from build123d import *

# Parameters (mm, degrees)
DOWELSUPPORT_DEPTH          = 1.905
DOWELSUPPORT_DEPTH_BACK     = 1.27
SKETCH3_R                   = 3.81
SKETCH5_W                   = 6.35
SKETCH5_H                   = 44.45
SLIDERDOWELSUPPORT_DEPTH    = 1.27
SKETCH17_R                  = 1.549999948
CUT_EXTRUDE1_DEPTH          = 19.685
CUT_EXTRUDE2_DEPTH          = 36.118212712
CUT_EXTRUDE2_DEPTH_BACK     = 36.118212712
SKETCH18_W                  = 1.27
SKETCH18_H                  = 25.4
LPATTERN1_COUNT             = 2
LPATTERN1_PITCH             = 25.4
LATERALSUPPORT_DEPTH        = 1.27
SKETCH8_W                   = 6.35
SKETCH8_H                   = 3
TABSUPPORT_DEPTH            = 1.27
STRINGDOWELSUPPORT_START    = -1.27
STRINGDOWELSUPPORT_DEPTH    = 5.715
INTERSUPPORT_DEPTH          = 1.27
SKETCH10_W                  = 6.35
SKETCH10_H                  = 3
TABBASE_DEPTH               = 1.27
SKETCH12_W                  = 6.35
SKETCH12_H                  = 3
TABDRAFT_DEPTH              = 1.73
TABDRAFT_DRAFT              = 5
TABDRAFT_PROFILE_2_DEPTH    = 1.73
TABDRAFT_PROFILE_2_DRAFT    = 5
STRINGDOWELHOLES_DEPTH      = 48.707819409
STRINGDOWELHOLES_DEPTH_BACK = 1.524
SKETCH14_R                  = 1.600000102
PULLEYDOWELHOLE_DEPTH       = 2.921
FILLET1_R                   = 6.35


with BuildPart() as part:
    # Sketch3 → DowelSupport (new, two sides: drawn at the far end of the back side and taken through both)
    with BuildSketch(Plane(origin=(0, 0, 0), x_dir=(0, 0, -1), z_dir=(1, 0, 0)).offset(-DOWELSUPPORT_DEPTH_BACK)):
        with Locations((0, 30.95625)):
            Circle(SKETCH3_R)
    extrude(amount=DOWELSUPPORT_DEPTH + DOWELSUPPORT_DEPTH_BACK)

    # Sketch8 → TabSupport (add, symmetric)
    with BuildSketch(Plane(origin=(0, 0, 0), x_dir=(0, 0, -1), z_dir=(1, 0, 0))):
        with Locations((0, 27.94)):
            Rectangle(SKETCH8_W, SKETCH8_H)
        with Locations((-12.7, 27.94)):
            Rectangle(SKETCH8_W, SKETCH8_H)
    extrude(amount=TABSUPPORT_DEPTH, both=True)


with BuildPart() as body_2:
    # Sketch5 → SliderDowelSupport (new, symmetric)
    with BuildSketch(Plane(origin=(0, 0, 0), x_dir=(0, 0, -1), z_dir=(1, 0, 0))):
        Rectangle(SKETCH5_W, SKETCH5_H)
    extrude(amount=SLIDERDOWELSUPPORT_DEPTH, both=True)

    # Sketch17 → Cut-Extrude1 (cut, symmetric)
    with BuildSketch(Plane(origin=(0, 0, 0), x_dir=(1, 0, 0), z_dir=(0, 1, 0))):
        with Locations((0.482000052, 0)):
            Circle(SKETCH17_R)
        with BuildLine():
            Line((2.032, 0), (2.032, 1.399999994))
            Line((2.032, 1.399999994), (1.147206678, 1.399999994))
            ThreePointArc((1.147206678, 1.399999994), (1.792261491, 0.828078983), (2.032, 0))
        make_face()
        with BuildLine():
            Line((2.032, -1.399999994), (2.032, 0))
            ThreePointArc((2.032, 0), (1.792261491, -0.828078983), (1.147206678, -1.399999994))
            Line((1.147206678, -1.399999994), (2.032, -1.399999994))
        make_face()
    extrude(amount=CUT_EXTRUDE1_DEPTH, both=True, mode=Mode.SUBTRACT)

    # Sketch18 → Cut-Extrude2 (cut, two sides: drawn at the far end of the back side and taken through both)
    with BuildSketch(Plane.ZY.offset(1.27).offset(-CUT_EXTRUDE2_DEPTH_BACK)):
        Rectangle(SKETCH18_W, SKETCH18_H)
    extrude(amount=CUT_EXTRUDE2_DEPTH + CUT_EXTRUDE2_DEPTH_BACK, mode=Mode.SUBTRACT)


with BuildPart() as lpattern1_1:
    # LPattern1: pattern copy
    add(body_2.part.moved(Location(Vector(0, 0, 1) * (1 * LPATTERN1_PITCH))))


with BuildPart() as body_4:
    # Sketch6 → LateralSupport (new, symmetric)
    with BuildSketch(Plane(origin=(0, 0, 0), x_dir=(0, 0, -1), z_dir=(1, 0, 0))):
        Polygon((7.392863577, 33.391434671), (5.805363577, 36.141065329), (8.169612929, 37.506065329), (9.523465192, 37.701124423), (10.602965192, 35.831375577), (9.757112929, 34.756434671), align=None)
    extrude(amount=LATERALSUPPORT_DEPTH, both=True)


with BuildPart() as tabsupport_piece_1:
    # of the separate pieces the step leaves, piece 1, a body of its own (tabsupport_pieces)
    add(part.part.solids().sort_by_distance((0, 30.95625, -3.81))[0])


with BuildPart() as tabsupport_piece_2:
    # of the separate pieces the step leaves, piece 2, a body of its own (tabsupport_pieces)
    add(part.part.solids().sort_by_distance((-1.27, 26.44, 9.525))[0])

    # Sketch15 → StringDowelSupport (add)
    with BuildSketch(Plane(origin=(0, 0, 0), x_dir=(0, 0, -1), z_dir=(1, 0, 0)).offset(STRINGDOWELSUPPORT_START)):
        with BuildLine():
            Line((-14.4145, 30.226), (-10.9855, 30.226))
            ThreePointArc((-10.9855, 30.226), (-8.6995, 27.94), (-10.9855, 25.654))
            Line((-10.9855, 25.654), (-14.4145, 25.654))
            ThreePointArc((-14.4145, 25.654), (-16.7005, 27.94), (-14.4145, 30.226))
        make_face()
    extrude(amount=STRINGDOWELSUPPORT_DEPTH)


with BuildPart() as body_2_1:
    add(body_2.part)

    add(lpattern1_1.part)  # InterSupport merges LPattern1_1

    add(body_4.part)  # InterSupport merges body 4

    add(tabsupport_piece_1.part)  # InterSupport merges TabSupport piece 1

    add(tabsupport_piece_2.part)  # InterSupport merges TabSupport piece 2
    # Sketch7 → InterSupport (add, symmetric)
    with BuildSketch(Plane(origin=(0, 0, 0), x_dir=(0, 0, -1), z_dir=(1, 0, 0))):
        Polygon((5.170363577, 37.240917591), (8.027863577, 32.291582409), (1.42875, 28.481582409), (-1.42875, 33.430917591), align=None)
        Polygon((-3.175, 15.875), (-3.175, 22.225), (3.175, 22.225), (3.175, 26.44), (0.923046602, 28.251940251), (-0.923046602, 33.660559749), (-10.9855, 30.226), (-14.4145, 30.226), (-15.109807039, 29.269115541), (-28.575, 22.225), (-22.225, 22.225), (-22.225, 0), (-3.175, 0), align=None)
    extrude(amount=INTERSUPPORT_DEPTH, both=True)

    # Sketch10 → TabBase (add)
    with BuildSketch(Plane.ZY.offset(1.27)):
        with Locations((0, 27.94)):
            Rectangle(SKETCH10_W, SKETCH10_H)
        with Locations((12.7, 27.94)):
            Rectangle(SKETCH10_W, SKETCH10_H)
    extrude(amount=TABBASE_DEPTH)


with BuildPart() as tabdraft_tool:
    # Sketch12 → TabDraft (with draft: the straight prism first)
    with BuildSketch(Plane.ZY.offset(2.54)):
        with Locations((0, 27.94)):
            Rectangle(SKETCH12_W, SKETCH12_H)
    extrude(amount=TABDRAFT_DEPTH)
    # TabDraft: the draft: its side faces are tilted about the plane it starts from
    tabdraft_sides = [tabdraft_tool.faces().sort_by_distance(p)[0] for p in [
        (-3.405, 27.94, 3.175),
        (-3.405, 29.44, 0),
        (-3.405, 27.94, -3.175),
        (-3.405, 26.44, 0),
    ]]
    draft(tabdraft_sides, Plane.ZY.offset(2.54), TABDRAFT_DRAFT)


with BuildPart() as body_2_2:
    add(body_2_1.part)

    # TabDraft: add tabdraft_tool
    add(tabdraft_tool.part)


with BuildPart() as tabdraft_profile_2_tool:
    # Sketch12 → TabDraft profile 2 (with draft: the straight prism first)
    with BuildSketch(Plane.ZY.offset(2.54)):
        with Locations((12.7, 27.94)):
            Rectangle(SKETCH12_W, SKETCH12_H)
    extrude(amount=TABDRAFT_PROFILE_2_DEPTH)
    # TabDraft profile 2: the draft: its side faces are tilted about the plane it starts from
    tabdraft_profile_2_sides = [tabdraft_profile_2_tool.faces().sort_by_distance(p)[0] for p in [
        (-3.405, 27.94, 9.525),
        (-3.405, 26.44, 12.7),
        (-3.405, 27.94, 15.875),
        (-3.405, 29.44, 12.7),
    ]]
    draft(tabdraft_profile_2_sides, Plane.ZY.offset(2.54), TABDRAFT_PROFILE_2_DRAFT)


with BuildPart() as body_2_3:
    add(body_2_2.part)

    # TabDraft profile 2: add tabdraft_profile_2_tool
    add(tabdraft_profile_2_tool.part)

    # Sketch16 → StringDowelHoles (cut, two sides: drawn at the far end of the back side and taken through both)
    with BuildSketch(Plane(origin=(1.905, 0, 0), x_dir=(0, 0, -1), z_dir=(1, 0, 0)).offset(-STRINGDOWELHOLES_DEPTH_BACK)):
        with BuildLine():
            Line((-13.00760401, 27.178), (-12.39239599, 27.178))
            ThreePointArc((-12.39239599, 27.178), (-9.385499898, 27.94), (-12.39239599, 28.702))
            Line((-12.39239599, 28.702), (-13.00760401, 28.702))
            ThreePointArc((-13.00760401, 28.702), (-16.014500102, 27.94), (-13.00760401, 27.178))
        make_face()
    extrude(amount=STRINGDOWELHOLES_DEPTH + STRINGDOWELHOLES_DEPTH_BACK, mode=Mode.SUBTRACT)

    # Sketch14 → PulleyDowelHole (cut)
    with BuildSketch(Plane(origin=(1.905, 0, 0), x_dir=(0, 0, -1), z_dir=(1, 0, 0))):
        with Locations((0, 30.95625)):
            Circle(SKETCH14_R)
    extrude(amount=-PULLEYDOWELHOLE_DEPTH, mode=Mode.SUBTRACT)

    # Mirror1: body 2 across plane


with BuildPart() as body_2_4:
    add(body_2_3.part)
    add(body_2_3.part.mirror(Plane.ZX))

    # Fillet1
    fillet1_edges = [body_2_4.edges().sort_by_distance(p)[0] for p in [
        (0, -22.225, 28.575),
        (0, 22.225, 28.575),
    ]]
    fillet(fillet1_edges, radius=FILLET1_R)


solid = body_2_4.part
Here's how the part is built. I have some questions about the finished solid (model axes, mm). A direction names the side the tool comes from. Give positions to 0.01 mm unless a question says otherwise; leave off trailing zeros. Loops run counter-clockwise (first coordinate to the right, second up) from the corner with the lowest first, then second, coordinate; pieces in that order, holes last. Notation, with made-up numbers: (-27, -33) -> (21, -33) arc R21 ccw to (21, -23) -> close; hole circle Ø11 at (-13, 25). An arc over 180 degrees is marked (long way). Answer as a JSON object with one key per item and string values. Group by question number.
Item 1: Imagine slicing it at C-C on x = -3.5. Write out the boundary of the cut face in (y, z).
Item 2: Thinking about a two-plate mould opening in Y: for faces 1 (the flat face through (0.018, -36.779, -10.056)), 2 (the flat face through (-3.393, 29.365, -0.044)), 3 (the cylindrical face through (2.18, -28.67, 16.58)), which applies, pulls with the +Y half, pulls with the -Y half, needs draft (parallel to the pull), parting line crosses it, or undercut?
Item 3: I need wall thicknesses on L1, parallel to Y at x = 1.1, z = 0 (3 decimals); L2, parallel to Z at x = 2.05, y = -27.94; L3, parallel to Z at x = 3.75, y = -29. Which ranges of each line are inside material? Lowest first, please.
Item 4: On a 3-axis mill with a long thin cutter (end or side, diameter ignored), from which of +Z, -Z, +X, -X, +Y, -Y can I reach the whole of each face in a straight line? I mean faces 4 (the flat face through (-3.4, -27.9, 9.6)), 5 (the flat face through (0.018, -34.083, -8.592)), 6 (the flat face through (0.018, -36.814, -6.971)), 7 (the flat face through (-3.393, 26.515, 12.656)), 8 (the flat face through (3, -25.654, 13)). Say none if no direction works.
Item 5: Imagine slicing it at D-D on z = 7.5. Write out the boundary of the cut face in (x, y), then the cut area to 3 significant figures.
Item 6: Imagine slicing it at A-A on y = 0. Write out the boundary of the cut face in (x, z) (3 decimals).
Item 7: Imagine slicing it at B-B on x = 3. Write out the boundary of the cut face in (y, z), then the cut area to 3 significant figures.
Item 8: Will these pins go through, and if not, where does the flat tip stop? pin 1 (1 mm diameter, centred on y = -31, z = 0.5, fed in from +X); pin 2 (10 mm diameter, centred on y = 28.5, z = 24.5, fed in from +X); pin 3 (2 mm diameter, centred on y = -10, z = 15.5, fed in from -X).
Answer list:
{
 "1": {"outline": "(-29.36, -3.09) -> (-26.52, -3.09) -> (-26.52, 3.09) -> (-29.36, 3.09) -> close; (-29.36, 9.61) -> (-26.52, 9.61) -> (-26.52, 15.79) -> (-29.36, 15.79) -> close; (26.52, -3.09) -> (29.36, -3.09) -> (29.36, 3.09) -> (26.52, 3.09) -> close; (26.52, 9.61) -> (29.36, 9.61) -> (29.36, 15.79) -> (26.52, 15.79) -> close"},
 "2": {"face 1": "pulls with the -Y half", "face 2": "pulls with the +Y half", "face 3": "undercut"},
 "3": {"L1": "y = -34.766 to -32.556, -29.356 to -19.685, 19.685 to 29.356, 32.556 to 34.766", "L2": "z = 8.7 to 9.39, 16.01 to 16.7", "L3": "z = 8.96 to 9.79, 12.18 to 13.22, 15.61 to 16.44"},
 "4": {"face 4": "-X, +Y, -Y", "face 5": "-Z, +X, -X", "face 6": "+X, -X, -Y", "face 7": "+Z, -Z, -X", "face 8": "+Z, -Z, +X"},
 "5": {"outline": "(-1.27, -31.42) -> (1.27, -31.42) -> (1.27, 31.42) -> (-1.27, 31.42) -> close", "area": "160 mm2"},
 "6": {"outline": "(-1.27, -3.175) -> (1.27, -3.175) -> (1.27, -1.4) -> (1.147, -1.4) arc R1.55 cw to (-0.932, -0.635) -> (-1.27, -0.635) -> close; (-1.27, 0.635) -> (-0.932, 0.635) arc R1.55 cw to (1.147, 1.4) -> (1.27, 1.4) -> (1.27, 24) -> (1.147, 24) arc R1.55 cw to (-0.932, 24.765) -> (-1.27, 24.765) -> close; (-1.27, 26.035) -> (-0.932, 26.035) arc R1.55 cw to (1.147, 26.8) -> (1.27, 26.8) -> (1.27, 28.575) -> (-1.27, 28.575) -> close"},
 "7": {"outline": "(-30.23, 10.99) arc R2.29 ccw to (-25.65, 10.99) -> (-25.65, 14.41) arc R2.29 ccw to (-30.23, 14.41) -> close; (25.65, 10.99) arc R2.29 ccw to (30.23, 10.99) -> (30.23, 14.41) arc R2.29 ccw to (25.65, 14.41) -> close; hole (-28.7, 12.39) arc R1.6 ccw (long way) to (-27.18, 12.39) -> (-27.18, 13.01) arc R1.6 ccw (long way) to (-28.7, 13.01) -> close; hole (27.18, 12.39) arc R1.6 ccw (long way) to (28.7, 12.39) -> (28.7, 13.01) arc R1.6 ccw (long way) to (27.18, 13.01) -> close", "area": "30.9 mm2"},
 "8": {"pin 1": "stops at x = -1.02", "pin 2": "stops at x = 1.27", "pin 3": "stops at x = -1.27"}
}
